```python
from build123d import *

# Parameters (mm, degrees)
SKETCH1_R           = 2.5
BOSS_EXTRUDE1_DEPTH = 8
REVOLVE1_ANGLE      = 180
CUT_EXTRUDE1_DEPTH  = 3


with BuildPart() as part:
    # Sketch1 → Boss-Extrude1 (new body)
    with BuildSketch(Plane(origin=(0, 0, 0), x_dir=(1, 0, 0), z_dir=(0, 1, 0))):
        Circle(SKETCH1_R)
    extrude(amount=BOSS_EXTRUDE1_DEPTH)

    # Sketch2 → Revolve1 (revolve)
    with BuildSketch(Plane(origin=(0, 8, 0), x_dir=(1, 0, 0), z_dir=(0, 1, 0))):
        with BuildLine():
            Line((0, 4), (0, -4))
            ThreePointArc((0, -4), (4, 0), (0, 4))
        make_face()
    revolve(axis=Axis((0, 8, -4), (0, 0, 1)), revolution_arc=REVOLVE1_ANGLE)

    # Sketch3 → Cut-Extrude1 (cut)
    with BuildSketch(Plane(origin=(0, 9, 0), x_dir=(1, 0, 0), z_dir=(0, 1, 0))):
        Polygon((0.5, 0.5), (5.630024771, 0.5), (5.630024771, -0.5), (0.5, -0.5), (0.5, -4.833323152), (-0.5, -4.833323152), (-0.5, -0.5), (-4.833323152, -0.5), (-4.833323152, 0.5), (-0.5, 0.5), (-0.5, 4.673982829), (0.5, 4.673982829), align=None)
    extrude(amount=CUT_EXTRUDE1_DEPTH, mode=Mode.SUBTRACT)


solid = part.part
```
Can you work these out from the model? Positions are in its coordinate system, mm. A direction names the side the tool comes from. Give positions to 0.01 mm unless a question says otherwise; leave off trailing zeros. Loops run counter-clockwise (first coordinate to the right, second up) from the corner with the lowest first, then second, coordinate; pieces in that order, holes last. Notation, with made-up numbers: M 54.25,33.5 L 97.25,33.5 A7 cw 97.25,45.5 Z; hole C 85.5,-38.75 d9. An arc over 180 degrees is marked long. Answer in a Markdown table with one row per item.
1. For pin 1 Ø2 at (x, y) = (-1.5, 3) entering from -Z; pin 2 Ø4 at (x, z) = (0.5, 2) entering from +Y; pin 3 Ø2.5 at (y, z) = (10.5, 3) entering from -X; pin 4 Ø3 at (x, y) = (3, 2.5) entering from +Z, each with a flat end and sliding along its axis, tell me the tip position at first contact or that it passes through.
Taken from the geometry:
| item | result |
|---|---|
| pin 1 | stops at z = -2.45 |
| pin 2 | stops at y = 11.94 |
| pin 3 | stops at x = -2.99 |
| pin 4 | stops at z = 2 |
2. Suppose I cut it at D-D on z = 2. Write out the boundary of the cut face in (x, y), plus the area to 3 significant figures.
Taken from the geometry:
| item | result |
|---|---|
| outline | M -3.46,8 L -1.5,8 L -1.5,0 L 1.5,0 L 1.5,8 L 3.46,8 A3.46 ccw 0.5,11.43 L 0.5,9 L -0.5,9 L -0.5,11.43 A3.46 ccw Z |
| area | 40.4 mm² |
3. Suppose I cut it at A-A on z = 0. Write out the boundary of the cut face in (x, y), plus the area to 3 significant figures.
Taken from the geometry:
| item | result |
|---|---|
| outline | M -4,8 L -2.5,8 L -2.5,0 L 2.5,0 L 2.5,8 L 4,8 A4 ccw 3.87,9 L -3.87,9 A4 ccw Z |
| area | 47.9 mm² |
4. Which directions (+Z, -Z, +X, -X, +Y, -Y) give clear straight access to the entire face, cutting with the end or side of a thin tool? Please do faces 1 (the flat face through (2, 10, -0.5)), 2 (the flat face through (2, 8, -2)), 3 (the flat face through (-0.5, 10, 2)).
Taken from the geometry:
| item | result |
|---|---|
| face 1 | +X, -X, +Y |
| face 2 | -Y |
| face 3 | +Z, -Z, +Y |
5. Thinking about a two-plate mould opening in Z: for faces 4 (the cylindrical face through (-0.54, 3.94, 2.44)), 5 (the flat face through (0, 9, 0)), 6 (the flat face through (0.5, 10, -2)), which applies, released by +Z, released by -Z, zero draft, split by the parting line, or undercut?
Taken from the geometry:
| item | result |
|---|---|
| face 4 | split by the parting line |
| face 5 | undercut |
| face 6 | zero draft |
6. Suppose I cut it at C-C on y = 1.5. Write out the boundary of the cut face in (x, z).
Taken from the geometry:
| item | result |
|---|---|
| outline | C 0,0 d5 |
7. If I drill on line 1 along X through (y, z) = (10.25, 3); line 2 along Y through (x, z) = (-3.5, 0); line 3 along Z through (x, y) = (-1.5, 1), over which ranges is the centre line in solid material (lowest first)?
Taken from the geometry:
| item | result |
|---|---|
| line 1 | x = -1.39 to -0.5, 0.5 to 1.39 |
| line 2 | y = 8 to 9 |
| line 3 | z = -2 to 2 |
8. Suppose I cut it at B-B on x = 0. Write out the boundary of the cut face in (y, z).
Taken from the geometry:
| item | result |
|---|---|
| outline | M 0,-2.5 L 8,-2.5 L 8,-4 A4 ccw 9,-3.87 L 9,3.87 A4 ccw 8,4 L 8,2.5 L 0,2.5 Z |
